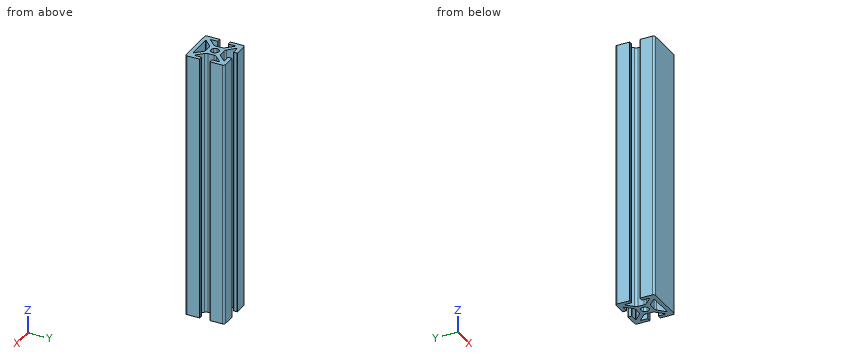
from build123d import *

# Parameters (mm, degrees)
BOSS_EXTRUDE1_DEPTH = 85.725
FILLET2_R           = 0.254
FILLET1_R           = 1.27
SKETCH5_W           = 7.112
SKETCH5_H           = 2.54
BOSS_EXTRUDE2_DEPTH = 171.45


with BuildPart() as part:
    # Sketch3 → Boss-Extrude1 (new body, symmetric)
    with BuildSketch(Plane.XY):
        with BuildLine():
            Line((-12.7, 12.7), (-1.796051224, 1.796051224))
            ThreePointArc((-1.796051224, 1.796051224), (-0.972015918, 2.346654013), (0, 2.54))
            Line((0, 2.54), (0, 4.826))
            Line((0, 4.826), (-1.977846327, 4.826))
            ThreePointArc((-1.977846327, 4.826), (-2.949862246, 5.019345987), (-3.773897552, 5.569948776))
            Line((-3.773897552, 5.569948776), (-7.772528286, 9.56857951))
            ThreePointArc((-7.772528286, 9.56857951), (-7.847628361, 9.946133082), (-7.527553898, 10.16))
            Line((-7.527553898, 10.16), (-3.302, 10.16))
            Line((-3.302, 10.16), (-3.302, 12.7))
            Line((-3.302, 12.7), (-12.7, 12.7))
        make_face()
    extrude(amount=BOSS_EXTRUDE1_DEPTH, both=True)

    # Fillet2
    fillet2_edges = [part.edges().sort_by_distance(p)[0] for p in [
        (-3.302, 12.7, 0),
        (-3.302, 10.16, 0),
    ]]
    fillet(fillet2_edges, radius=FILLET2_R)

    # Mirror1: part across plane


with BuildPart() as part_1:
    add(part.part)
    add(part.part.mirror(Plane(origin=(0, 0, 85.725), x_dir=(0, 0, 1), z_dir=(0.707106781, 0.707106781, 0))))

    # Fillet1
    fillet1_edges = [part_1.edges().sort_by_distance(p)[0] for p in [
        (-12.7, 12.7, 0),
    ]]
    fillet(fillet1_edges, radius=FILLET1_R)

    # Mirror2: part across plane


with BuildPart() as part_2:
    add(part_1.part)
    add(part_1.part.mirror(Plane(origin=(0, 0, 85.725), x_dir=(0, 0, 1), z_dir=(0, 1, 0))))

    # Mirror5: part across plane


with BuildPart() as part_3:
    add(part_2.part)
    add(part_2.part.mirror(Plane(origin=(0, 0, 85.725), x_dir=(0, 0, 1), z_dir=(-1, 0, 0))))

    # Sketch5 → Boss-Extrude2 (add, through all)
    with BuildSketch(Plane.XY.offset(85.725)):
        with Locations((0, -11.43)):
            Rectangle(SKETCH5_W, SKETCH5_H)
    extrude(amount=-BOSS_EXTRUDE2_DEPTH)


solid = part_3.part
The model under review builds one solid part; all positions refer to its coordinate system, in mm. Coordinates: 2 decimals unless noted, no trailing zeros.
(1) Wall thickness on L1, parallel to Y at x = -7.25, z = 38.5; L2, parallel to X at y = -6.5, z = -67; L3, parallel to X at y = -4.25, z = -56: over which ranges is each line inside the solid? List them lowest first.
Determined:
L1: y = -12.7 to -10.16, -9.05 to -5.45, 5.45 to 9.05, 10.16 to 12.7
L2: x = -12.7 to -10.16, -8.3 to -4.7, 4.7 to 8.3, 10.16 to 12.7
L3: x = -12.7 to -10.16, -6.05 to 6.05, 10.16 to 12.7
(2) Insertion check: P1, Ø1.2, axis at y = -1, z = 9, coming from the -X side; P2, Ø1.5, axis at y = -1, z = 16, coming from the +X side; P3, Ø0.6, axis at x = 12, z = 2.5, coming from the +Y side. Each pin has a flat end and moves straight along its axis. Give the tip position at first contact, or say it passes through.
Determined:
P1: stops at x = -4.83
P2: stops at x = 4.83
P3: stops at y = 12.67
(3) Consider section A-A, the plane z = 25.5. Give the number of separate pieces and of enclosed holes in the cut face, plus the area to 3 significant figures.
Determined:
separate pieces: 1
enclosed holes: 2
area: 332 mm2
